Source: CAD feature listing. Evaluate the final solid. Frame: model axes, mm. Face numbers are marked on the shaded views. A direction names the side the tool comes from. Round coordinates to 2 decimals unless told otherwise and drop trailing zeros. Loops run counter-clockwise (first coordinate to the right, second up) from the corner with the lowest first, then second, coordinate; pieces in that order, holes last. Notation, with made-up numbers: M 87.25,-37 L 112.25,-37 A12 cw 112.25,-20 Z; hole C 16,32.5 d4. An arc over 180 degrees is marked long. One line per item, written item: value.
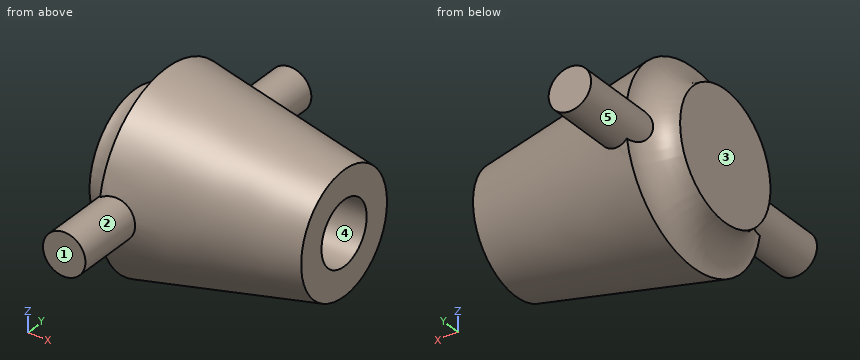
Autodesk Inventor part; units mm, degrees
ref_plane "YZ Plane" through (0, 0, 0) normal (1, 0, 0) x (0, 1, 0)
ref_plane "XZ Plane" through (0, 0, 0) normal (0, 1, 0) x (-1, 0, 0)
ref_plane "XY Plane" through (0, 0, 0) normal (0, 0, 1) x (1, 0, 0)
sketch "Sketch1" plane through (0, 0, 0) normal (0, 0, 1) x (1, 0, 0)
  line L0 (87.63, 0) -> (112.6819, 0)
  line L1 (112.6819, 0) -> (112.6819, 7.239)
  line L2 (112.6819, 7.239) -> (91.44, 11.43)
  line L3 (87.63, 11.43) -> (87.63, 7.62) construction
  line L4 (85.09, -8.9952) -> (85.09, 8.9952)
  line L5 (85.09, 0) -> (87.63, 0) construction
  arc A0 (91.44, 11.43) -> (87.63, 7.62) centre (87.63, 11.43) ccw construction
  arc A1 (87.63, 7.62) -> (91.44, 11.43) centre (87.63, 11.43) ccw
  line L6 (87.63, 7.62) -> (87.63, 0)
  line L7 (91.44, 11.43) -> (87.63, 11.43) construction
  point P0 (0, 0)
  dimension "d0" = 25.4
  dimension "d1" = 11.43
  dimension "d2" = 2.54
  dimension "d3" = 7.62
  dimension "d5" = 7.239
revolve "Revolution1" add sketch "Sketch1" angle 360 about axis through (87.63, 0, 0) along (1, 0, 0)
sketch "Sketch2" plane through (0, 0, 0) normal (0, 1, 0) x (-1, 0, 0)
  circle A0 centre (-92.71, 0) radius 2.54
  circle A1 centre (-92.71, 0) radius 2.54
  circle A2 centre (-92.71, 0) radius 2.54
  circle A3 centre (-92.71, 0) radius 2.54
  circle A4 centre (-92.71, 0) radius 2.54
  point P0 (0, 0)
extrude "Extrusion1" add sketch "Sketch2" along normal mid plane 38.1
sketch "Sketch3" plane through (112.6819, 0, 0) normal (1, 0, 0) x (0, 0, -1)
  circle A0 centre (0, 0) radius 3.81
  dimension "d8" = 7.62
extrude "Extrusion2" cut sketch "Sketch3" against normal blind 12.7
properties part number "Arm_Wheel_Attachment"
1. Section query C-C (z = 0). Return the cut outline in (x, y), and give its area (3 significant figures).
Report:
outline: M 87.63,-7.62 A3.81 cw 90.17,-8.59 L 90.17,-19.05 L 95.25,-19.05 L 95.25,-10.68 L 112.68,-7.24 L 112.68,-3.81 L 99.98,-3.81 L 99.98,3.81 L 112.68,3.81 L 112.68,7.24 L 95.25,10.68 L 95.25,19.05 L 90.17,19.05 L 90.17,8.59 A3.81 cw 87.63,7.62 Z
area: 449 mm2
2. Section query D-D (x = 92.71). Return the cut outline in (y, z).
Report:
outline: M -19.05,-2.54 L -10.89,-2.54 A11.18 ccw 10.89,-2.54 L 19.05,-2.54 L 19.05,2.54 L 10.89,2.54 A11.18 ccw -10.89,2.54 L -19.05,2.54 Z
3. Section query B-B (x = 104.5). Return the cut outline in (y, z).
Report:
outline: C 0,0 d17.71; hole C 0,0 d7.62
4. Pin query (flat end, axial travel): pin 1 (2 mm diameter, centred on y = -5, z = -8, fed in from -X); pin 2 (2 mm diameter, centred on x = 92.5, y = 9, fed in from +Z); pin 3 (12 mm diameter, centred on x = 100, y = -8, fed in from -Z). Return the tip coordinate at first contact, or that it passes through.
Report:
pin 1: stops at x = 89.98
pin 2: stops at z = 7.91
pin 3: stops at z = -9.95
5. Ray query, line 1 (Y direction, x = 105.75, z = -2.5); line 2 (Y direction, x = 104.5, z = 0.5); line 3 (X direction, y = -0.5, z = -3). Return the intervals inside material, ascending. Write a range as [from, to].
Report:
line 1: y = [-8.24, -2.88], [2.88, 8.24]
line 2: y = [-8.84, -3.78], [3.78, 8.84]
line 3: x = [87.63, 99.98]
6. Section query A-A (y = 0). Return the cut outline in (x, z), and give its area (3 significant figures).
Report:
outline: M 87.63,-7.62 A3.81 cw 91.44,-11.43 L 112.68,-7.24 L 112.68,-3.81 L 99.98,-3.81 L 99.98,3.81 L 112.68,3.81 L 112.68,7.24 L 91.44,11.43 A3.81 cw 87.63,7.62 Z
area: 364 mm2
7. Reachability of the marked faces 1, 2, 3, 4 and 5 from +Z, -Z, +X, -X, +Y, -Y: full face, straight path, thin tool, end or side. Return the list, or none.
Report:
face 1: +Z, -Z, +X, -X, -Y
face 2: -Y
face 3: +Z, -Z, -X, +Y, -Y
face 4: +X
face 5: +Y
